The model under review builds one solid part; all positions refer to its coordinate system, in mm. Give positions to 0.01 mm unless a question says otherwise; leave off trailing zeros. Order: outer loops, then holes, each group sorted by start corner. A loop starts at its lowest first (then second) coordinate and runs counter-clockwise, first axis right, second up.
```python
from build123d import *

# Parameters (mm, degrees)
Y_KSEKLIK_EKSTR_ZYON1_DEPTH = 40
BO_ALTMA1_T                 = -3
Y_KSEKLIK_EKSTR_ZYON2_START = -3
Y_KSEKLIK_EKSTR_ZYON2_DEPTH = 3


with BuildPart() as part:
    # Çizim1 → Yükseklik-Ekstrüzyon1 (new body)
    with BuildSketch(Plane.XY):
        with BuildLine():
            Line((-90, 50), (90, 50))
            ThreePointArc((90, 50), (93.535533906, 48.535533906), (95, 45))
            Line((95, 45), (95, -45))
            ThreePointArc((95, -45), (93.535533906, -48.535533906), (90, -50))
            Line((90, -50), (-90, -50))
            ThreePointArc((-90, -50), (-93.535533906, -48.535533906), (-95, -45))
            Line((-95, -45), (-95, 45))
            ThreePointArc((-95, 45), (-93.535533906, 48.535533906), (-90, 50))
        make_face()
    extrude(amount=Y_KSEKLIK_EKSTR_ZYON1_DEPTH)

    # İç Boşaltma1
    bo_altma1_openings = [part.faces().sort_by_distance(p)[0] for p in [
        (0, 0, 40),
    ]]
    offset(amount=BO_ALTMA1_T, openings=bo_altma1_openings, kind=Kind.INTERSECTION)

    # Çizim2 → Yükseklik-Ekstrüzyon2 (add)
    with BuildSketch(Plane.XY.offset(40).offset(Y_KSEKLIK_EKSTR_ZYON2_START)):
        with BuildLine():
            Line((90, 47), (-90, 47))
            ThreePointArc((-90, 47), (-91.414213562, 46.414213562), (-92, 45))
            Line((-92, 45), (-92, -45))
            ThreePointArc((-92, -45), (-91.414213562, -46.414213562), (-90, -47))
            Line((-90, -47), (90, -47))
            ThreePointArc((90, -47), (91.414213562, -46.414213562), (92, -45))
            Line((92, -45), (92, 45))
            ThreePointArc((92, 45), (91.414213562, 46.414213562), (90, 47))
        make_face()
    extrude(amount=Y_KSEKLIK_EKSTR_ZYON2_DEPTH)


solid = part.part
```
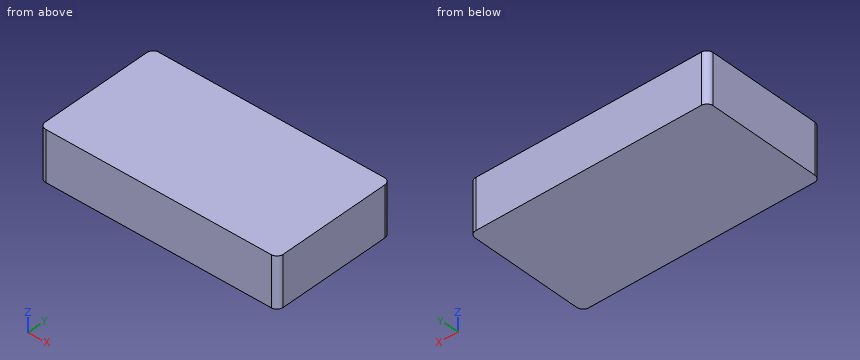
Item 1: Clearance check with a flat-ended pin moving along its axis: pin 1 Ø1.5 at (x, y) = (-37, 8) entering from -Z. State where the tip first meets the part, or that it passes through.
Values found:
pin 1: stops at z = 0
Item 2: Take a section at C-C (x = 2). Give the boundary of the cut face in (y, z), and give its area (3 significant figures).
Values found:
outline: (-50, 0) - (50, 0) - (50, 40) - (-50, 40) - close; hole (-47, 3) - (47, 3) - (47, 37) - (-47, 37) - close
area: 804 mm2
Item 3: Take a section at B-B (y = 34). Give the boundary of the cut face in (x, z), and give its area (3 significant figures).
Values found:
outline: (-95, 0) - (95, 0) - (95, 40) - (-95, 40) - close; hole (-92, 3) - (92, 3) - (92, 37) - (-92, 37) - close
area: 1,340 mm2
Item 4: Take a section at A-A (z = 26). Give the boundary of the cut face in (x, y).
Values found:
outline: (-95, -45) arc R5 ccw to (-90, -50) - (90, -50) arc R5 ccw to (95, -45) - (95, 45) arc R5 ccw to (90, 50) - (-90, 50) arc R5 ccw to (-95, 45) - close; hole (-92, -45) arc R2 ccw to (-90, -47) - (90, -47) arc R2 ccw to (92, -45) - (92, 45) arc R2 ccw to (90, 47) - (-90, 47) arc R2 ccw to (-92, 45) - close
Item 5: For line 1 (Z direction, x = -62, y = -34); line 2 (Y direction, x = -35, z = 10); line 3 (X direction, y = -20.5, z = 29.5), list the stretches that pass through material, from the lowest coordinate up.
Values found:
line 1: z = 0 to 3, 37 to 40
line 2: y = -50 to -47, 47 to 50
line 3: x = -95 to -92, 92 to 95
